The drawing under review shows one solid part. Ordinate dimensions are in mm from its lowest x, y, z. A direction names the side the tool comes from. Coordinates: 2 decimals unless noted, no trailing zeros. Order: outer loops, then holes, each group sorted by start corner. A loop starts at its lowest first (then second) coordinate and runs counter-clockwise, first axis right, second up.
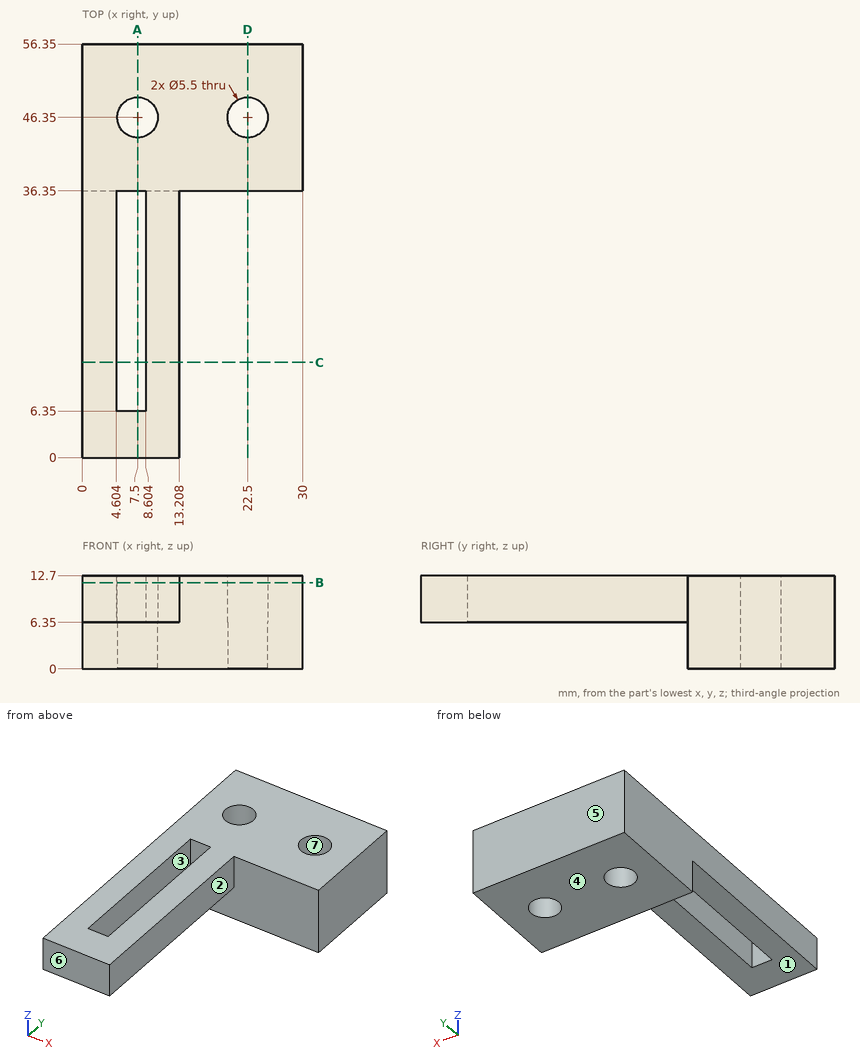
(1) For pin 1 Ø3 at (y, z) = (14.5, 9) entering from +X; pin 2 Ø5 at (x, y) = (22.5, 46.35) entering from -Z; pin 3 Ø10.5 at (x, y) = (7.5, 19.5) entering from -Z, all flat-tipped, find the tip position at first contact; note any pin that passes through.
A:
pin 1: stops at x = 13.21
pin 2: passes through
pin 3: stops at z = 6.35
(2) We need section A-A, the plane x = 7.5. Write out the cut boundary in (y, z), and give its area (3 significant figures).
A:
outline: (0, 6.35) - (6.35, 6.35) - (6.35, 12.7) - (0, 12.7) - close; (36.35, 0) - (43.6, 0) - (43.6, 12.7) - (36.35, 12.7) - close; (49.1, 0) - (56.35, 0) - (56.35, 12.7) - (49.1, 12.7) - close
area: 224 mm2
(3) We need section B-B, the plane z = 11.75. Write out the cut boundary in (x, y).
A:
outline: (0, 0) - (13.21, 0) - (13.21, 36.35) - (30, 36.35) - (30, 56.35) - (0, 56.35) - close; hole (4.6, 6.35) - (8.6, 6.35) - (8.6, 36.35) - (4.6, 36.35) - close; hole circle Ø5.5 at (7.5, 46.35); hole circle Ø5.5 at (22.5, 46.35)
(4) Wall thickness on probe 1 along X at (y, z) = (46.35, 3.5); probe 2 along Y at (x, z) = (7.5, 7.5); probe 3 along Y at (x, z) = (22.5, 8.75): over which ranges is each line inside the solid? List them lowest first.
A:
probe 1: x = 0 to 4.75, 10.25 to 19.75, 25.25 to 30
probe 2: y = 0 to 6.35, 36.35 to 43.6, 49.1 to 56.35
probe 3: y = 36.35 to 43.6, 49.1 to 56.35
(5) We need section C-C, the plane y = 13. Write out the cut boundary in (x, z).
A:
outline: (0, 6.35) - (4.6, 6.35) - (4.6, 12.7) - (0, 12.7) - close; (8.6, 6.35) - (13.21, 6.35) - (13.21, 12.7) - (8.6, 12.7) - close
(6) We need section D-D, the plane x = 22.5. Write out the cut boundary in (y, z), and give its area (3 significant figures).
A:
outline: (36.35, 0) - (43.6, 0) - (43.6, 12.7) - (36.35, 12.7) - close; (49.1, 0) - (56.35, 0) - (56.35, 12.7) - (49.1, 12.7) - close
area: 184 mm2
(7) Machinability: for the marked faces 1, 2 and 3, which of the approach directions +Z, -Z, +X, -X, +Y, -Y give a long, thin tool a straight path to every point of the face, cutting with its end or side? Answer none if there is none.
A:
face 1: -Z, +X, -X, -Y
face 2: +Z, -Z, +X, -Y
face 3: +Z, -Z
(8) Draft analysis for pull direction Y (two halves, no side actions). For the marked faces 4, 5, 6 and 7, state which applies: released by +Y, released by -Y, zero draft, split by the parting line, or undercut.
A:
face 4: zero draft
face 5: released by +Y
face 6: released by -Y
face 7: undercut
